Answer from the drawing. Dimensions are ordinates in mm from the lowest x, y and z of the part. A direction names the side the tool comes from. Round coordinates to 2 decimals unless told otherwise and drop trailing zeros. Write each loop counter-clockwise with the first axis right and the second up, starting at its lowest first coordinate (ties: lowest second). Pieces come first, ordered by that corner, then holes. Notation, with made-up numbers: (-21.75, 57.25) - (35.25, 57.25) arc R22 cw to (35.25, 88.25) - close; hole circle Ø6 at (47.5, -6). An arc over 180 degrees is marked (long way). Write item = value, one per line. Start each with the question number.
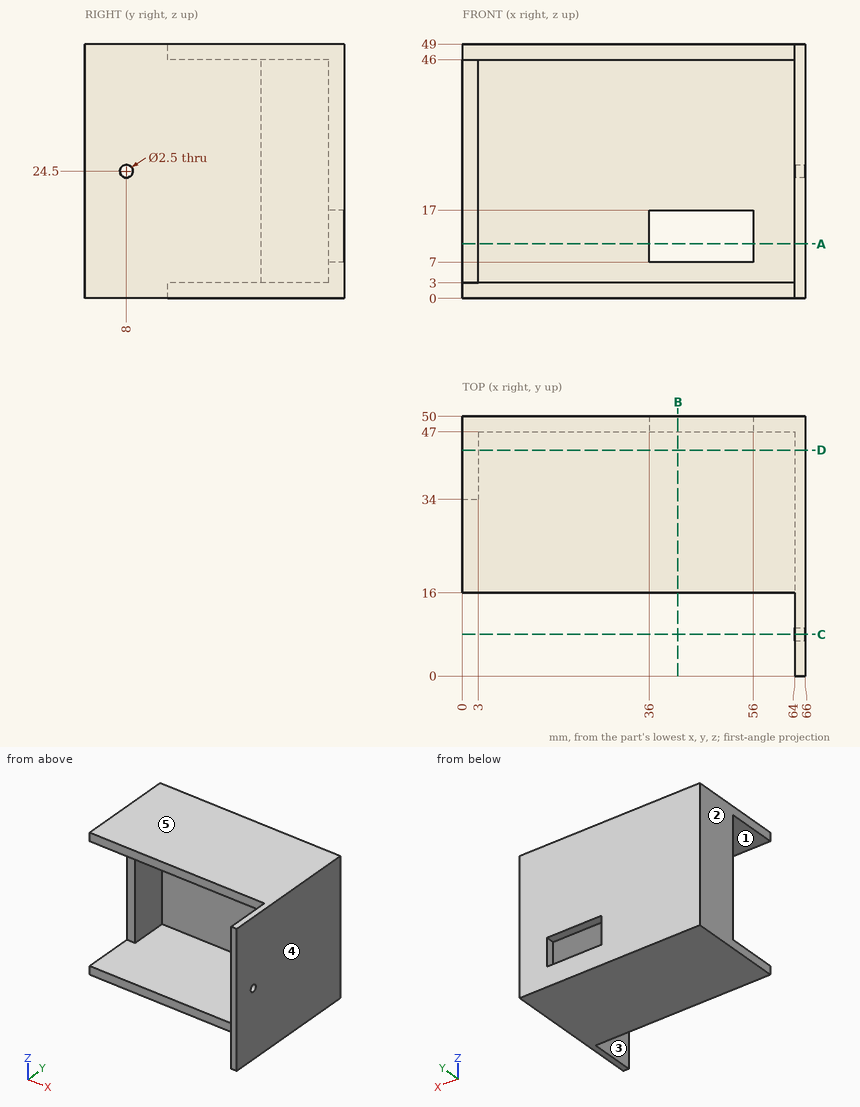
1. For a pull along X with two mould halves and no side action, classify the marked faces 3, 4 and 5 as released by +X, released by -X, zero draft, split by the parting line, or undercut.
2. Consider line 1 (Y direction, x = 65.5, z = 24.5); line 2 (Z direction, x = 64.45, y = 8); line 3 (Z direction, x = 34, y = 41). Determine where each line is inside the solid, lowest interval first.
3. Find section C-C on y = 8. Give the vertices of the cut face in (x, z).
4. Find section D-D on y = 43.5. Give the vertices of the cut face in (x, z), plus the area to 3 significant figures.
5. Find section A-A on z = 10.5. Give the vertices of the cut face in (x, y).
6. Which of the six approach directions +Z, -Z, +X, -X, +Y, -Y give full straight-line access (tool end or side, diameter ignored) to the marked faces 1 and 2?
7. Find section B-B on x = 41.5. Give the vertices of the cut face in (y, z), plus the area to 3 significant figures.
8. Each of these flat-tipped pins is pushed along its axis until it touches: pin 1 (0.9 mm diameter, centred on x = 1.5, z = 23.5, fed in from -Y); pin 2 (2.5 mm diameter, centred on x = 22, z = 1.5, fed in from -Y); pin 3 (4 mm diameter, centred on x = 10, z = 6, fed in from -Y); pin 4 (1.5 mm diameter, centred on y = 8, z = 24.5, fed in from +X). Where does it stop, or does it pass through?
Answer key:
q1.face_3 = undercut
q1.face_4 = released by +X
q1.face_5 = zero draft
q2.line_1 = 0 to 6.75, 9.25 to 50
q2.line_2 = 0 to 23.25, 25.75 to 49
q2.line_3 = 0 to 3, 46 to 49
q3.outline = (64, 0) - (66, 0) - (66, 23.25) - (64, 23.25) - close; (64, 25.75) - (66, 25.75) - (66, 49) - (64, 49) - close
q4.outline = (0, 0) - (66, 0) - (66, 49) - (0, 49) - close; hole (3, 3) - (64, 3) - (64, 46) - (3, 46) - close
q4.area = 611 mm²
q5.outline = (0, 34) - (3, 34) - (3, 47) - (36, 47) - (36, 50) - (0, 50) - close; (56, 47) - (64, 47) - (64, 0) - (66, 0) - (66, 50) - (56, 50) - close
q6.face_1 = -Y
q6.face_2 = +Z, -Z, -X, +Y, -Y
q7.outline = (16, 0) - (50, 0) - (50, 7) - (47, 7) - (47, 3) - (16, 3) - close; (16, 46) - (47, 46) - (47, 17) - (50, 17) - (50, 49) - (16, 49) - close
q7.area = 303 mm²
q8.pin_1 = 34
q8.pin_2 = 16
q8.pin_3 = 47
q8.pin_4 = through
